Answer from the drawing. Dimensions are ordinates in mm from the lowest x, y and z of the part. Give positions to 0.01 mm unless a question says otherwise; leave off trailing zeros. Order: outer loops, then holes, each group sorted by start corner. A loop starts at its lowest first (then second) coordinate and runs counter-clockwise, first axis right, second up. Notation, with made-up numbers: M -20.5,-6 L 36.5,-6 A20 cw 36.5,21 Z; hole C 23.5,-25.5 d4. An arc over 180 degrees is marked long. One line per item, written item: value.
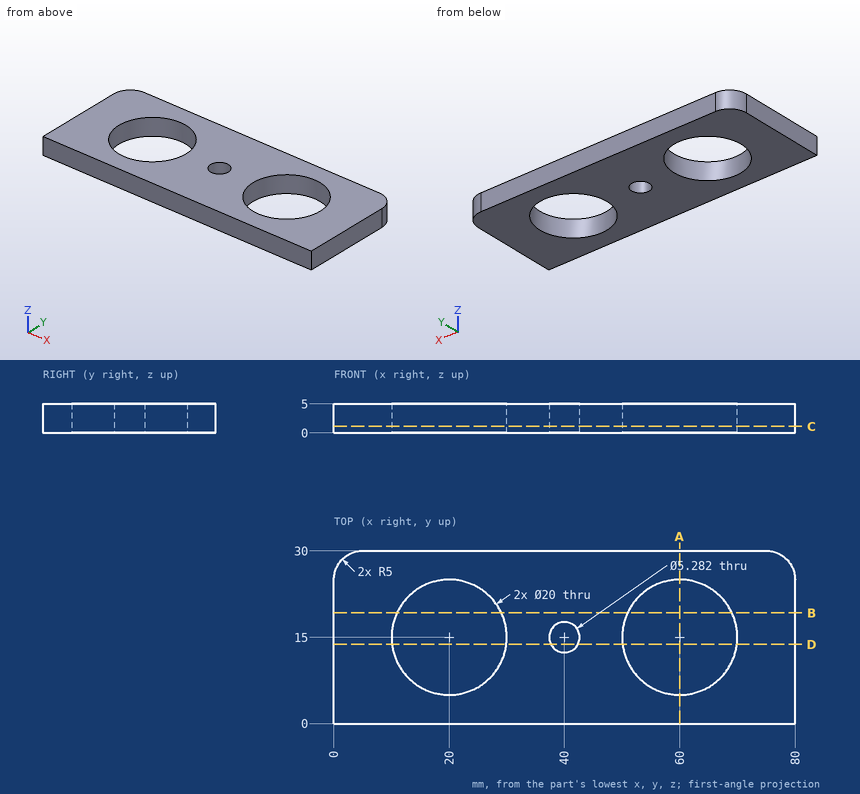
(1) Given P1, Ø1, axis at x = 59, y = 5.5, coming from the +Z side, flat-ended and moving along its own axis, determine where the tip first touches the part or whether it passes through.
Findings:
P1: stops at z = 5
(2) Find the intervals of material crossed by probe 1 along Y at (x, z) = (60, 1.6); probe 2 along X at (y, z) = (22, 3.9); probe 3 along Y at (x, z) = (40, 2.85), in increasing order. Write a range as from..to.
Findings:
probe 1: y = 0..5, 25..30
probe 2: x = 0..12.86, 27.14..52.86, 67.14..80
probe 3: y = 0..12.36, 17.64..30
(3) Section C-C, the plane z = 1.1 is taken. Give the vertices of the cut face in (x, y), then the cut area to 3 significant figures.
Findings:
outline: M 0,0 L 80,0 L 80,25 A5 ccw 75,30 L 5,30 A5 ccw 0,25 Z; hole C 20,15 d20; hole C 40,15 d5.28; hole C 60,15 d20
area: 1,740 mm^2
(4) Section A-A, the plane x = 60 is taken. Give the vertices of the cut face in (y, z), then the cut area to 3 significant figures.
Findings:
outline: M 0,0 L 5,0 L 5,5 L 0,5 Z; M 25,0 L 30,0 L 30,5 L 25,5 Z
area: 50.0 mm^2
(5) Section B-B, the plane y = 19.25 is taken. Give the vertices of the cut face in (x, z).
Findings:
outline: M 0,0 L 10.95,0 L 10.95,5 L 0,5 Z; M 29.05,0 L 50.95,0 L 50.95,5 L 29.05,5 Z; M 69.05,0 L 80,0 L 80,5 L 69.05,5 Z
(6) Section D-D, the plane y = 13.75 is taken. Give the vertices of the cut face in (x, z).
Findings:
outline: M 0,0 L 10.08,0 L 10.08,5 L 0,5 Z; M 29.92,0 L 37.67,0 L 37.67,5 L 29.92,5 Z; M 42.33,0 L 50.08,0 L 50.08,5 L 42.33,5 Z; M 69.92,0 L 80,0 L 80,5 L 69.92,5 Z
